```python
from build123d import *

# Parameters (mm, degrees)
F4_R     = 115.5
F4_R_2   = 112.5
F2_DEPTH = 25
F3_R     = 37.5
F5_DEPTH = 2


with BuildPart() as f1:
    # F0 (on Front) → F1 (revolve)
    with BuildSketch(Plane.XZ):
        Polygon((0, -71.573662), (0, 296.426338), (-45.129046, 341.555384), (-135, 341.555384), (-135, 339.555384), (-45.957473, 339.555384), (-2, 295.597911), (-2, -71.037763), (-11.177422, -86.933525), (-135, -86.933525), (-135, -88.933525), (-10.022722, -88.933525), align=None)
    revolve(axis=Axis((-135, 0, 126.31093), (0, 0, -1)))

    # F4 (on face) → F2 (join, symmetric)
    with BuildSketch(Plane.XY.offset(341.555384)):
        with Locations((-135, 0)):
            Circle(F4_R)
        with Locations((-135, 0)):
            Circle(F4_R_2, mode=Mode.SUBTRACT)
    extrude(amount=F2_DEPTH, both=True)

    # F3 (on face) → F5 (cut, through all)
    with BuildSketch(Plane.XY.offset(341.555384)):
        with Locations((-141.725168, -27.080007)):
            Circle(F3_R)
    extrude(amount=-F5_DEPTH, mode=Mode.SUBTRACT)


solid = f1.part
```
Could you check a few things on this model? Use its own coordinates, in mm. A direction names the side the tool comes from. Round coordinates to 2 decimals unless told otherwise and drop trailing zeros. Loops run counter-clockwise (first coordinate to the right, second up) from the corner with the lowest first, then second, coordinate; pieces in that order, holes last. Notation, with made-up numbers: M -12,19.5 L 26,19.5 A16 ccw 26,23.5 Z; hole C -25,54.5 d9. An arc over 180 degrees is marked long. Answer as CSV lines item,"result".
1) If I drill on probe 1 along Y at (x, z) = (-134.5, 99); probe 2 along Z at (x, y) = (-164.5, 59); probe 3 along Y at (x, z) = (-142.5, 332), over which ranges is the centre line in solid material (lowest first)?
From the geometry:
probe 1,"-135 to -133, 133 to 135"
probe 2,"-88.93 to -86.93, 339.56 to 341.56"
probe 3,"-115.26 to -112.25, -99.14 to -96.31, 96.31 to 99.14, 112.25 to 115.26"
2) Imagine slicing it at A-A on z = 143. List the corners of the cut face in (x, y) for me.
From the geometry:
outline,"C -135,0 d270; hole C -135,0 d266"
3) Which directions (+Z, -Z, +X, -X, +Y, -Y) give clear straight access to the entire face, cutting with the end or side of a thin tool? Please do faces 1 (the flat face through (-24, -25, 366.555)), 2 (the flat face through (-134, 19, 339.555)), 3 (the flat face through (-136, 19, 341.555)).
From the geometry:
face 1,"+Z, +X, -X, +Y, -Y"
face 2,"none"
face 3,"+Z"
4) We'd pull the mould along Y, two halves only. Please class faces 4 (the conical face through (-154.899, 89.61, 336.806)), 5 (the cylindrical face through (-250.39, 5.08, 341.91)), 6 (the flat face through (-133, -2, -88.934)): released by +Y, released by -Y, zero draft, split by the parting line, or undercut.
From the geometry:
face 4,"undercut"
face 5,"split by the parting line"
face 6,"zero draft"
5) For pin 1 Ø10 at (x, y) = (-44, 96.5) entering from +Z; pin 2 Ø3 at (y, z) = (107, 305.5) entering from -X; pin 3 Ø10 at (x, z) = (-188, -25.5) entering from +Y, each with a flat end and sliding along its axis, tell me the tip position at first contact or that it passes through.
From the geometry:
pin 1,"z = 303.79"
pin 2,"x = -205.03"
pin 3,"y = 126.18"
